from build123d import *

# Parameters (mm, degrees)
SKETCH1_R                      = 10
BOSS_EXTRUDE1_DEPTH            = 32.5
BOSS_EXTRUDE2_DEPTH            = 2
F_2_8_2_8_DIAMETER_HOLE1_D     = 2.8
F_2_8_2_8_DIAMETER_HOLE1_DEPTH = 70
F_2_8_2_8_DIAMETER_HOLE1_TIP   = 0.841204867
SKETCH5_R                      = 4
BOSS_EXTRUDE3_DEPTH            = 2
SKETCH6_R                      = 2
BOSS_EXTRUDE4_DEPTH            = 8


with BuildPart() as part:
    # Sketch1 → Boss-Extrude1 (new body)
    with BuildSketch(Plane(origin=(0, 0, 0), x_dir=(0, 0, -1), z_dir=(1, 0, 0))):
        Circle(SKETCH1_R)
    extrude(amount=BOSS_EXTRUDE1_DEPTH)

    # Sketch2 → Boss-Extrude2 (add)
    with BuildSketch(Plane.ZY):
        with BuildLine():
            Line((-12.5, 3), (12.5, 3))
            ThreePointArc((12.5, 3), (15.5, 0), (12.5, -3))
            Line((12.5, -3), (-12.5, -3))
            ThreePointArc((-12.5, -3), (-15.5, 0), (-12.5, 3))
        make_face()
    extrude(amount=BOSS_EXTRUDE2_DEPTH)

    # Ø2.8 (2.8) Diameter Hole1
    with Locations(Plane.ZY.offset(2)):
        with Locations((-12.5, 0), (12.5, 0)):
            Hole(F_2_8_2_8_DIAMETER_HOLE1_D / 2, depth=F_2_8_2_8_DIAMETER_HOLE1_DEPTH)
            with Locations((0, 0, -(F_2_8_2_8_DIAMETER_HOLE1_DEPTH + F_2_8_2_8_DIAMETER_HOLE1_TIP / 2))):  # 118° drill point
                Cone(0, F_2_8_2_8_DIAMETER_HOLE1_D / 2, F_2_8_2_8_DIAMETER_HOLE1_TIP, mode=Mode.SUBTRACT)

    # Sketch5 → Boss-Extrude3 (add)
    with BuildSketch(Plane.ZY.offset(2)):
        with Locations(Location((0, 0, 0), (0, 0, 228.590377891))):
            Circle(SKETCH5_R)
    extrude(amount=BOSS_EXTRUDE3_DEPTH)

    # Sketch6 → Boss-Extrude4 (add)
    with BuildSketch(Plane.ZY.offset(4)):
        Circle(SKETCH6_R)
    extrude(amount=BOSS_EXTRUDE4_DEPTH)


solid = part.part
Read the model definition and answer for the solid it produces. Units are mm, in the model's axes. A direction names the side the tool comes from. Coordinates: 2 decimals unless noted, no trailing zeros. Loops run counter-clockwise (first coordinate to the right, second up) from the corner with the lowest first, then second, coordinate; pieces in that order, holes last.
Q1. The part is cut by section D-D on y = 8. Write down the section's boundary in (x, z), and give its area (3 significant figures).
Q2. The part is cut by section A-A on y = 0. Write down the section's boundary in (x, z), and give its area (3 significant figures).
Q3. Consider probe 1 along Y at (x, z) = (-0.9, 12.5); probe 2 along X at (y, z) = (-5.5, -6.5); probe 3 along X at (y, z) = (-2.25, 6). Determine where each line is inside the solid, lowest interval first.
Q4. Each of these flat-tipped pins is pushed along its axis until it touches: pin 1 Ø6.5 at (y, z) = (1, 12) entering from -X; pin 2 Ø3.5 at (y, z) = (7.5, -4.5) entering from -X; pin 3 Ø1.5 at (x, z) = (7, -1) entering from +Y. Where does it stop, or does it pass through?
Q5. The part is cut by section C-C on x = 17. Write down the section's boundary in (y, z), and give its area (3 significant figures).
Q6. The mould has two halves that part along X. Classify faces 5 (the face through (0, -1, 11)), 6 (the face through (-1, -0.1, -15.5)), 7 (the face through (-1, -3, 0)): +X half, -X half, draft (parallel to the pull), parting line (faces both ways), or undercut.
Q7. The part is cut by section B-B on z = 0. Write down the section's boundary in (x, y), and give its area (3 significant figures).
Q8. Which of the six approach directions +Z, -Z, +X, -X, +Y, -Y give full straight-line access (tool end or side, diameter ignored) to faces 1 (the face through (-1, 3, 0)), 2 (the face through (-2.986, -3.656, -1.622)), 3 (the face through (-0.99, 0.06, 13.9)), 4 (the face through (-2, -3.4, 0.1))?
Results below:
1. outline: (0, -6) - (32.5, -6) - (32.5, 6) - (0, 6) - close
1. area: 390 mm2
2. outline: (-12, -2) - (-4, -2) - (-4, -4) - (-2, -4) - (-2, -11.1) - (0, -11.1) - (0, -10) - (32.5, -10) - (32.5, 10) - (0, 10) - (0, 11.1) - (-2, 11.1) - (-2, 4) - (-4, 4) - (-4, 2) - (-12, 2) - close; (-2, -15.5) - (0, -15.5) - (0, -13.9) - (-2, -13.9) - close; (-2, 13.9) - (0, 13.9) - (0, 15.5) - (-2, 15.5) - close
2. area: 749 mm2
3. probe 1: y = -3 to -1.4, 1.4 to 3
3. probe 2: x = 0 to 32.5
3. probe 3: x = -2 to 32.5
4. pin 1: stops at x = -2
4. pin 2: stops at x = 0
4. pin 3: stops at y = 10
5. outline: circle Ø20 at (0, 0)
5. area: 314 mm2
6. face 5: +X half
6. face 6: draft
6. face 7: undercut
7. outline: (-12, -2) - (-4, -2) - (-4, -4) - (-2, -4) - (-2, -3) - (0, -3) - (0, -10) - (32.5, -10) - (32.5, 10) - (0, 10) - (0, 3) - (-2, 3) - (-2, 4) - (-4, 4) - (-4, 2) - (-12, 2) - close
7. area: 710 mm2
8. face 1: +Z, -Z, +Y
8. face 2: -X
8. face 3: +X, -X
8. face 4: +Z, -Z, -Y
